Could you check a few things on this model? Use its own coordinates, in mm. Face numbers are marked on the shaded views. A direction names the side the tool comes from. Coordinates: 2 decimals unless noted, no trailing zeros. Write each loop counter-clockwise with the first axis right and the second up, starting at its lowest first coordinate (ties: lowest second). Pieces come first, ordered by that corner, then holes.
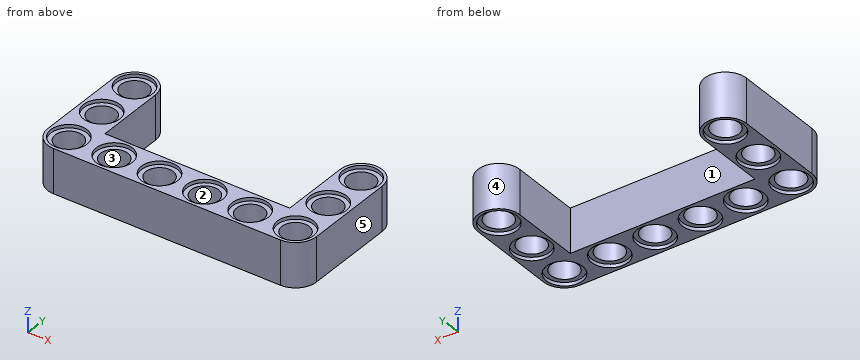
```python
from build123d import *

# Parameters (mm, degrees)
F0_R     = 2.4
F1_DEPTH = 7.8
F2_R     = 3.2
F3_DEPTH = 0.6
F4_R     = 3.2
F5_DEPTH = 0.6


with BuildPart() as f1:
    # F0 (on Top) → F1 (new body)
    with BuildSketch(Plane.XY):
        with BuildLine():
            ThreePointArc((-3.7, 3.7), (-2.616295, 1.083705), (0, 0))
            Line((0, 0), (40, 0))
            ThreePointArc((40, 0), (42.616295, 1.083705), (43.7, 3.7))
            ThreePointArc((43.7, 3.7), (42.616295, 6.316295), (40, 7.4))
            Line((40, 7.4), (36.3, 7.4))
            Line((36.3, 7.4), (3.7, 7.4))
            Line((3.7, 7.4), (3.7, 19.7))
            ThreePointArc((3.7, 19.7), (0, 23.4), (-3.7, 19.7))
            Line((-3.7, 19.7), (-3.7, 3.7))
        make_face()
        with Locations((0, 3.7)):
            Circle(F0_R, mode=Mode.SUBTRACT)
        with Locations((8, 3.7)):
            Circle(F0_R, mode=Mode.SUBTRACT)
        with Locations((16, 3.7)):
            Circle(F0_R, mode=Mode.SUBTRACT)
        with Locations((24, 3.7)):
            Circle(F0_R, mode=Mode.SUBTRACT)
        with Locations((32, 3.7)):
            Circle(F0_R, mode=Mode.SUBTRACT)
        with Locations((40, 3.7)):
            Circle(F0_R, mode=Mode.SUBTRACT)
        with Locations((0, 11.7)):
            Circle(F0_R, mode=Mode.SUBTRACT)
        with Locations((0, 19.7)):
            Circle(F0_R, mode=Mode.SUBTRACT)
        with BuildLine():
            ThreePointArc((40, 7.4), (42.616295, 6.316295), (43.7, 3.7))
            Line((43.7, 3.7), (43.7, 19.7))
            ThreePointArc((43.7, 19.7), (40, 23.4), (36.3, 19.7))
            Line((36.3, 19.7), (36.3, 7.4))
            Line((36.3, 7.4), (40, 7.4))
        make_face()
        with Locations((40, 11.7)):
            Circle(F0_R, mode=Mode.SUBTRACT)
        with Locations((40, 19.7)):
            Circle(F0_R, mode=Mode.SUBTRACT)
    extrude(amount=F1_DEPTH)

    # F2 (on face) → F3 (cut)
    with BuildSketch(Plane.XY.offset(7.8)):
        with Locations((0, 3.7)):
            Circle(F2_R)
        with Locations((8, 3.7)):
            Circle(F2_R)
        with Locations((16, 3.7)):
            Circle(F2_R)
        with Locations((24, 3.7)):
            Circle(F2_R)
        with Locations((32, 3.7)):
            Circle(F2_R)
        with Locations((40, 3.7)):
            Circle(F2_R)
        with Locations((0, 11.7)):
            Circle(F2_R)
        with Locations((40, 11.7)):
            Circle(F2_R)
        with Locations((0, 19.7)):
            Circle(F2_R)
        with Locations((40, 19.7)):
            Circle(F2_R)
    extrude(amount=-F3_DEPTH, mode=Mode.SUBTRACT)

    # F4 (on face) → F5 (cut)
    with BuildSketch(Plane(origin=(0, 0, 0), x_dir=(1, 0, 0), z_dir=(0, 0, -1))):
        with Locations((0, -11.7)):
            Circle(F4_R)
        with Locations((0, -3.7)):
            Circle(F4_R)
        with Locations((8, -3.7)):
            Circle(F4_R)
        with Locations((16, -3.7)):
            Circle(F4_R)
        with Locations((24, -3.7)):
            Circle(F4_R)
        with Locations((32, -3.7)):
            Circle(F4_R)
        with Locations((40, -3.7)):
            Circle(F4_R)
        with Locations((40, -11.7)):
            Circle(F4_R)
        with Locations((0, -19.7)):
            Circle(F4_R)
        with Locations((40, -19.7)):
            Circle(F4_R)
    extrude(amount=-F5_DEPTH, mode=Mode.SUBTRACT)


solid = f1.part
```
1. On a 3-axis mill with a long thin cutter (end or side, diameter ignored), from which of +Z, -Z, +X, -X, +Y, -Y can I reach the whole of each face in a straight line? I mean the marked faces 1 and 2. Say none if no direction works.
Verdict:
face 1: +Z, -Z, +Y
face 2: +Z, -Z
2. I want a section at B-B on x = 16. Please give me the cut outline in (y, z).
Verdict:
outline: (0, 0) - (0.5, 0) - (0.5, 0.6) - (1.3, 0.6) - (1.3, 7.2) - (0.5, 7.2) - (0.5, 7.8) - (0, 7.8) - close; (6.1, 0.6) - (6.9, 0.6) - (6.9, 0) - (7.4, 0) - (7.4, 7.8) - (6.9, 7.8) - (6.9, 7.2) - (6.1, 7.2) - close
3. Please list where these lines run through material, in increasing order: line 1 along X through (y, z) = (19.7, 3); line 2 along Y through (x, z) = (0, 2.75); line 3 along Y through (x, z) = (16, 0.2).
Verdict:
line 1: x = -3.7 to -2.4, 2.4 to 3.7, 36.3 to 37.6, 42.4 to 43.7
line 2: y = 0 to 1.3, 6.1 to 9.3, 14.1 to 17.3, 22.1 to 23.4
line 3: y = 0 to 0.5, 6.9 to 7.4
4. If we mould it in two halves opening along Y, with no side actions, what happens to the marked faces 3, 4 and 5? For each: pulls with the +Y half, pulls with the -Y half, needs draft (parallel to the pull), parting line crosses it, or undercut.
Verdict:
face 3: undercut
face 4: pulls with the +Y half
face 5: needs draft
5. I want a section at A-A on y = 11.7. Give the number of separate pieces and of enclosed holes in the cut face, plus the area to 3 significant figures.
Verdict:
separate pieces: 4
enclosed holes: 0
area: 36.7 mm2
6. For pin 1 (3 mm diameter, centred on x = 33, z = 3, fed in from +Y); pin 2 (1.9 mm diameter, centred on x = 15, y = 3, fed in from -Z); pin 3 (6 mm diameter, centred on x = 0, y = 19.7, fed in from +Z); pin 4 (1.9 mm diameter, centred on x = 1, y = 2.5, fed in from -Z), each with a flat end and sliding along its axis, tell me the tip position at first contact or that it passes through.
Verdict:
pin 1: stops at y = 7.4
pin 2: passes through
pin 3: stops at z = 7.2
pin 4: stops at z = 0.6
7. I want a section at D-D on x = 7.5. Please give me the cut outline in (y, z).
Verdict:
outline: (0, 0) - (0.54, 0) - (0.54, 0.6) - (1.35, 0.6) - (1.35, 7.2) - (0.54, 7.2) - (0.54, 7.8) - (0, 7.8) - close; (6.05, 0.6) - (6.86, 0.6) - (6.86, 0) - (7.4, 0) - (7.4, 7.8) - (6.86, 7.8) - (6.86, 7.2) - (6.05, 7.2) - close
